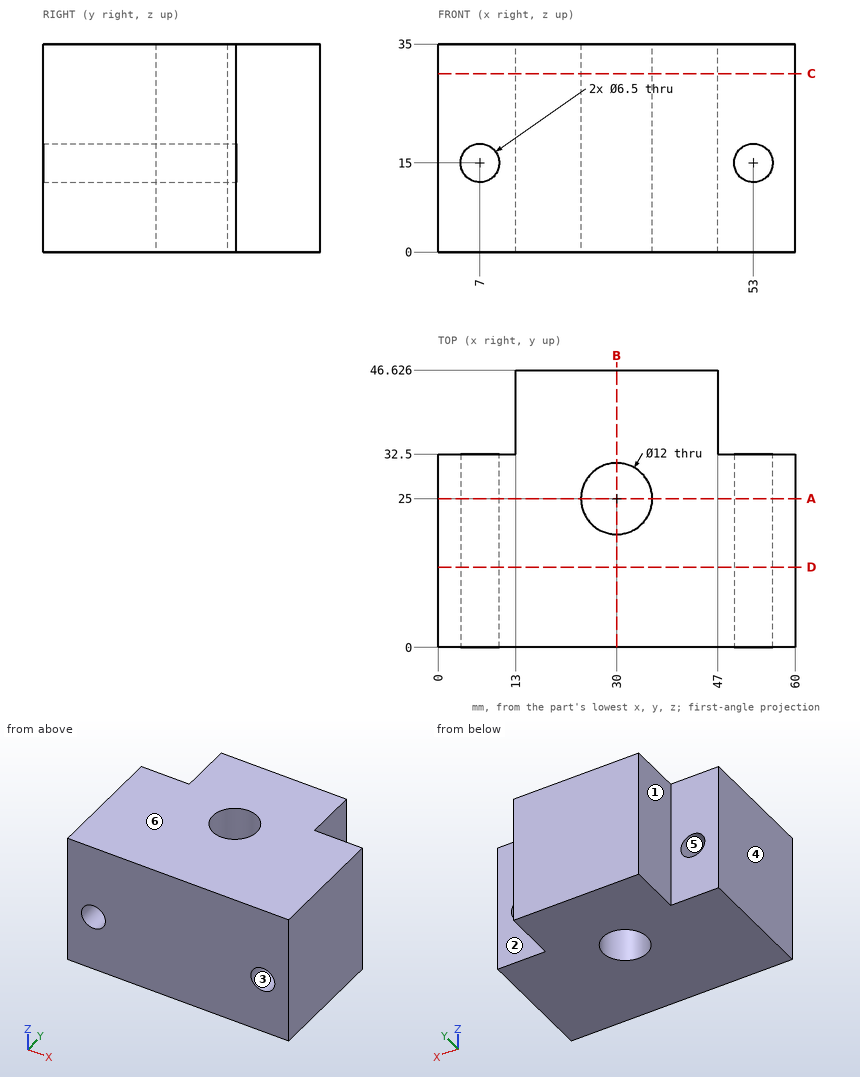
Verification items for this drawing (mm, ordinates from the low corner). A direction names the side the tool comes from. Coordinates: 2 decimals unless noted, no trailing zeros. Order: outer loops, then holes, each group sorted by start corner. A loop starts at its lowest first (then second) coordinate and runs counter-clockwise, first axis right, second up. Notation, with made-up numbers: (23, 76.25) -> (35, 76.25) arc R33 cw to (35, 112.25) -> close; hole circle Ø11 at (-7.5, 33.25). An arc over 180 degrees is marked (long way). Put each result on its own line as item: value. Start each with the question number.
1. Go/stop test with flat-tipped pins: pin 1 Ø6.5 at (x, z) = (7.5, 22) entering from +Y; pin 2 Ø11.5 at (y, z) = (41.5, 13) entering from -X; pin 3 Ø4 at (y, z) = (35.5, 24) entering from +X. Record where each tip stops, or that it passes through.
2. Material ranges on L1, parallel to Z at x = 53, y = 19; L2, parallel to Y at x = 30, z = 18.5 (1 decimal); L3, parallel to X at y = 14.5, z = 13, recorded low to high. Write a range as [from, to].
3. Cross-section at A-A, the plane y = 25. Record the boundary of the cut face in (x, z), then the cut area to 3 significant figures.
4. Cross-section at B-B, the plane x = 30. Record the boundary of the cut face in (y, z) (1 decimal).
5. Cross-section at C-C, the plane z = 30. Record the boundary of the cut face in (x, y) (1 decimal).
6. Cross-section at D-D, the plane y = 13.5. Record the boundary of the cut face in (x, z).
7. Mould release check, pull along X, two halves, no side actions. Record for the marked faces 4, 5 and 6: released by +X, released by -X, zero draft, split by the parting line, or undercut.
8. Access from +Z, -Z, +X, -X, +Y, -Y to the whole of each face (thin tool, end or side, straight path). Record for the marked faces 1, 2 and 3.
Computed:
1. pin 1: y = 32.5
1. pin 2: x = 13
1. pin 3: x = 47
2. L1: [0, 11.75], [18.25, 35]
2. L2: [0, 19], [31, 46.6]
2. L3: [0, 4.44], [9.56, 50.44], [55.56, 60]
3. outline: (0, 0) -> (24, 0) -> (24, 35) -> (0, 35) -> close; (36, 0) -> (60, 0) -> (60, 35) -> (36, 35) -> close; hole circle Ø6.5 at (7, 15); hole circle Ø6.5 at (53, 15)
3. area: 1,610 mm2
4. outline: (0, 0) -> (19, 0) -> (19, 35) -> (0, 35) -> close; (31, 0) -> (46.6, 0) -> (46.6, 35) -> (31, 35) -> close
5. outline: (0, 0) -> (60, 0) -> (60, 32.5) -> (47, 32.5) -> (47, 46.6) -> (13, 46.6) -> (13, 32.5) -> (0, 32.5) -> close; hole circle Ø12 at (30, 25)
6. outline: (0, 0) -> (60, 0) -> (60, 35) -> (0, 35) -> close; hole circle Ø6.5 at (7, 15); hole circle Ø6.5 at (53, 15)
7. face 4: released by -X
7. face 5: undercut
7. face 6: zero draft
8. face 1: +Z, -Z, -X, +Y
8. face 2: +Z, -Z, +X, +Y
8. face 3: +Y, -Y
